Could you check a few things on this model? Use its own coordinates, in mm. A direction names the side the tool comes from. Coordinates: 2 decimals unless noted, no trailing zeros. Loops run counter-clockwise (first coordinate to the right, second up) from the corner with the lowest first, then second, coordinate; pieces in that order, holes last. Notation, with made-up numbers: M 78.5,-30.75 L 87.5,-30.75 A5 ccw 87.5,-21.75 Z; hole C 19,-23.75 d10. An arc over 180 degrees is marked long. Write each question's results on one line, items separated by ' | '.
```python
from build123d import *


with BuildPart() as part:
    # 스케치1 → 회전1 (revolve)
    with BuildSketch(Plane.XY, mode=Mode.PRIVATE) as revolve_1_sk:
        Polygon((10, 0), (19, 0), (19, 20), (20, 20), (20, 45), (12.5, 115), (10, 115), (10, 85), (5, 85), (5, 80), (7.782730507, 80), (7.782730507, 75.813819554), (10, 70.553192673), align=None)
    revolve(revolve_1_sk.sketch.rotate(Axis((0, 0, 0), (0, 1, 0)), 90), axis=Axis((0, 0, 0), (0, 1, 0)))


solid = part.part
```
(1) Imagine slicing it at C-C, the plane y = 8.5. List the corners of the cut face in (x, z) for me, and give its area (3 significant figures).
Reported:
outline: C 0,0 d38; hole C 0,0 d20 | area: 820 mm2
(2) Imagine slicing it at D-D, the plane y = 94. List the corners of the cut face in (x, z) for me, and give its area (3 significant figures).
Reported:
outline: C 0,0 d29.5; hole C 0,0 d20 | area: 369 mm2
(3) Imagine slicing it at B-B, the plane z = 0. List the corners of the cut face in (x, y) for me, and give its area (3 significant figures).
Reported:
outline: M -20,20 L -19,20 L -19,0 L -10,0 L -10,70.55 L -7.78,75.81 L -7.78,80 L -5,80 L -5,85 L -10,85 L -10,115 L -12.5,115 L -20,45 Z; M 5,80 L 7.78,80 L 7.78,75.81 L 10,70.55 L 10,0 L 19,0 L 19,20 L 20,20 L 20,45 L 12.5,115 L 10,115 L 10,85 L 5,85 Z | area: 1,820 mm2
(4) Imagine slicing it at A-A, the plane x = 0. List the corners of the cut face in (y, z) for me.
Reported:
outline: M 0,-19 L 20,-19 L 20,-20 L 45,-20 L 115,-12.5 L 115,-10 L 85,-10 L 85,-5 L 80,-5 L 80,-7.78 L 75.81,-7.78 L 70.55,-10 L 0,-10 Z; M 0,10 L 70.55,10 L 75.81,7.78 L 80,7.78 L 80,5 L 85,5 L 85,10 L 115,10 L 115,12.5 L 45,20 L 20,20 L 20,19 L 0,19 Z
(5) Please list where these lines run through material, in increasing order: probe 1 along Z at (x, y) = (3, 15); probe 2 along Z at (x, y) = (2, 97.5); probe 3 along X at (y, z) = (77.85, 0). Write a range as from..to.
Reported:
probe 1: z = -18.76..-9.54, 9.54..18.76 | probe 2: z = -14.24..-9.8, 9.8..14.24 | probe 3: x = -16.48..-7.78, 7.78..16.48
(6) Will these pins go through, and if not, where does the flat tip stop? P1, Ø3, axis at y = 31, z = -5.5, coming from the -X side; P2, Ø4, axis at x = 9, y = 39, coming from the +Z side (3 decimals); P3, Ø1.5, axis at y = 61, z = -4.5, coming from the +X side; P4, Ø4.5, axis at x = -0.5, z = -0.5, coming from the -Y side.
Reported:
P1: stops at x = -19.6 | P2: stops at z = 18.735 | P3: stops at x = 17.92 | P4: passes through
(7) Which directions (+Z, -Z, +X, -X, +Y, -Y) give clear straight access to the entire face, cutting with the end or side of a thin tool? Please do faces 4 (the flat face through (7, 20, 18)), 5 (the cylindrical face through (0, 82, 5)), 6 (the flat face through (-5, 85, -2)).
Reported:
face 4: -Y | face 5: +Y, -Y | face 6: +Y
(8) If we mould it in two halves opening along X, with no side actions, what happens to faces 1 (the conical face through (-16.06, 80.49, 2.11)), 2 (the flat face through (8, 0, 8)), 3 (the cylindrical face through (0, 100, 10))? For each: released by +X, released by -X, zero draft, split by the parting line, or undercut.
Reported:
face 1: split by the parting line | face 2: zero draft | face 3: undercut
